Could you check a few things on this model? Use its own coordinates, in mm. A direction names the side the tool comes from. Coordinates: 2 decimals unless noted, no trailing zeros. Loops run counter-clockwise (first coordinate to the right, second up) from the corner with the lowest first, then second, coordinate; pieces in that order, holes last. Notation, with made-up numbers: M -26,81 L 6,81 A16 cw 6,95 Z; hole C -37,-23 d3. An arc over 180 degrees is marked long. Write each question's results on one line, items separated by ' | '.
```python
from build123d import *

# Parameters (mm, degrees)
SKETCH_R        = 6.3
PAD_DEPTH       = 20
SKETCH001_R     = 4.3
PAD001_DEPTH    = 6
SKETCH002_W     = 1.8
SKETCH002_H     = 1.7
SKETCH002_W_2   = 1.4
SKETCH002_H_2   = 1.9
SKETCH002_W_3   = 1.7
POCKET_DEPTH    = 5.99
SKETCH003_R     = 4.5
POCKET001_DEPTH = 7
SKETCH004_W     = 1.3
SKETCH004_H     = 1.5
SKETCH004_W_2   = 1.5
SKETCH004_H_2   = 1.3
PAD002_DEPTH    = 7
SKETCH005_R     = 1.5
POCKET002_DEPTH = 50


with BuildPart() as part:
    # Sketch → Pad (new body)
    with BuildSketch(Plane.XY):
        with Locations((7, 7)):
            Circle(SKETCH_R)
    extrude(amount=PAD_DEPTH)

    # Sketch001 (on Face3 of Pad) → Pad001 (join)
    with BuildSketch(Plane.XY.offset(20)):
        with Locations((7, 7)):
            Circle(SKETCH001_R)
    extrude(amount=PAD001_DEPTH)

    # Sketch002 (on Face5 of Pad001) → Pocket (cut)
    with BuildSketch(Plane.XY.offset(26)):
        with Locations((7, 11.15)):
            Rectangle(SKETCH002_W, SKETCH002_H)
        with Locations((7, 2.85)):
            Rectangle(SKETCH002_W, SKETCH002_H)
        with Locations((3, 7.05)):
            Rectangle(SKETCH002_W_2, SKETCH002_H_2)
        with Locations((11.15, 7.05)):
            Rectangle(SKETCH002_W_3, SKETCH002_H_2)
    extrude(amount=-POCKET_DEPTH, mode=Mode.SUBTRACT)

    # Sketch003 (on Face2 of Pocket) → Pocket001 (cut)
    with BuildSketch(Plane(origin=(0, 0, 0), x_dir=(1, 0, 0), z_dir=(0, 0, -1))):
        with Locations((7, -7)):
            Circle(SKETCH003_R)
    extrude(amount=-POCKET001_DEPTH, mode=Mode.SUBTRACT)

    # Sketch004 (on Face6 of Pocket001) → Pad002 (join)
    with BuildSketch(Plane(origin=(0, 0, 7), x_dir=(1, 0, 0), z_dir=(0, 0, -1))):
        with Locations((7, -2.9)):
            Rectangle(SKETCH004_W, SKETCH004_H)
        with Locations((7, -11.1)):
            Rectangle(SKETCH004_W, SKETCH004_H)
        with Locations((11.1, -7)):
            Rectangle(SKETCH004_W_2, SKETCH004_H_2)
        with Locations((2.9, -7)):
            Rectangle(SKETCH004_W_2, SKETCH004_H_2)
    extrude(amount=PAD002_DEPTH)

    # Sketch005 (on Face28 of Pad002) → Pocket002 (cut)
    with BuildSketch(Plane.XY.offset(26)):
        with Locations((7, 7)):
            Circle(SKETCH005_R)
    extrude(amount=-POCKET002_DEPTH, mode=Mode.SUBTRACT)


solid = part.part
```
(1) Imagine slicing it at D-D, the plane x = 4. List the corners of the cut face in (y, z) for me, and give its area (3 significant figures).
Reported:
outline: M 1.46,0 L 3.65,0 L 3.65,7 L 10.35,7 L 10.35,0 L 12.54,0 L 12.54,20 L 10.08,20 L 10.08,26 L 3.92,26 L 3.92,20 L 1.46,20 Z | area: 212 mm2
(2) Will these pins go through, and if not, where does the flat tip stop? P1, Ø0.6, axis at y = 3, z = 3.5, coming from the -X side; P2, Ø3, axis at y = 7.5, z = 10.5, coming from the -X side; P3, Ø4, axis at x = 3, z = 14, coming from the +Y side; P4, Ø1, axis at y = 7, z = 24, coming from the -X side.
Reported:
P1: stops at x = 1.9 | P2: stops at x = 0.7 | P3: stops at y = 12.97 | P4: stops at x = 3.7
(3) If we mould it in two halves opening along Y, with no side actions, what happens to faces 6 (the flat face through (7, 10.3, 23)), 7 (the cylindrical face through (3.79, 10.153, 3.451)), 8 (the flat face through (11, 4, 20))? For each: released by +Y, released by -Y, zero draft, split by the parting line, or undercut.
Reported:
face 6: released by +Y | face 7: undercut | face 8: zero draft
(4) Please list where these lines run through material, in increasing order: probe 1 along Y at (x, z) = (7, 16.75); probe 2 along Y at (x, z) = (7, 21.25); probe 3 along X at (y, z) = (7.75, 24). Write a range as from..to.
Reported:
probe 1: y = 0.7..5.5, 8.5..13.3 | probe 2: y = 3.7..5.5, 8.5..10.3 | probe 3: x = 3.7..5.7, 8.3..10.3
(5) Which directions (+Z, -Z, +X, -X, +Y, -Y) give clear straight access to the entire face, cutting with the end or side of a thin tool? Please do faces 1 (the flat face through (7.9, 3, 23)), 2 (the flat face through (3, 6.1, 23)), 3 (the flat face through (3, 7.65, 4)), 4 (the flat face through (7.9, 11, 23)), 5 (the flat face through (10.3, 7, 23)).
Reported:
face 1: +Z, -Y | face 2: +Z, -X | face 3: -Z | face 4: +Z, +Y | face 5: +Z, +X
(6) Imagine slicing it at C-C, the plane z = 21.5. List the corners of the cut face in (x, y) for me, and give its area (3 significant figures).
Reported:
outline: M 2.8,6.1 A4.3 ccw 6.1,2.8 L 6.1,3.7 L 7.9,3.7 L 7.9,2.8 A4.3 ccw 11.2,6.1 L 10.3,6.1 L 10.3,8 L 11.18,8 A4.3 ccw 7.9,11.2 L 7.9,10.3 L 6.1,10.3 L 6.1,11.2 A4.3 ccw 2.82,8 L 3.7,8 L 3.7,6.1 Z; hole C 7,7 d3 | area: 43.9 mm2
